Check sheet for the modelled part. Datum: model origin and axes. Units: mm. A direction names the side the tool comes from. Give positions to 0.01 mm unless a question says otherwise; leave off trailing zeros. Loops run counter-clockwise (first coordinate to the right, second up) from the corner with the lowest first, then second, coordinate; pieces in that order, holes last. Notation, with made-up numbers: (33, -11) -> (88, -11) arc R24 cw to (88, 12) -> close; hole circle Ø10 at (-26.75, -28.5). An arc over 180 degrees is marked (long way). Write each question's results on one line, items separated by ' | '. Start each with the question number.
1. Gauge pin test, flat ends, axial feed: pin 1 Ø6 at (y, z) = (21.5, 4) entering from +X; pin 2 Ø2.5 at (x, z) = (29, 7.5) entering from +Y; pin 3 Ø2 at (y, z) = (1, 10) entering from -X. Record the tip position at first contact, or that the pin passes through.
2. Cross-section at B-B on y = -11.25. Record the boundary of the cut face in (x, z), and give its area (3 significant figures).
3. Cross-section at C-C on x = 22.5. Record the boundary of the cut face in (y, z).
4. Cross-section at A-A on x = -40. Record the boundary of the cut face in (y, z), and give its area (3 significant figures).
5. Cross-section at D-D on y = -24. Record the boundary of the cut face in (x, z), and give its area (3 significant figures).
6. Tool access check on faces 5 (the face through (26, 1.25, 8)), 6 (the face through (27, 5.85, 5)), 7 (the face through (-40, -13, 2)), 8 (the face through (36, -13, 4)), 9 (the face through (42.747, -23.267, 7.379)). Record the directions out of +Z, -Z, +X, -X, +Y, -Y that give a thin tool (end or side, any length) a straight path to the whole face; none if there is none.
7. Mould release check, pull along X, two halves, no side actions. Record for faces 1 (the face through (34, -7, 7)), 2 (the face through (35.005, -15.662, 7.28)), 3 (the face through (1, -28, 7)), 4 (the face through (-25.08, 19.38, 7.4)): +X half, -X half, draft (parallel to the pull), parting line (faces both ways), or undercut.
8. Material ranges on L1, parallel to X at y = -10.5, z = 11.75; L2, parallel to Y at x = 22, z = 7.5; L3, parallel to Y at x = 0, z = 11.5, recorded low to high. Write a range as from..to.
from build123d import *

# Parameters (mm, degrees)
SKETCH1_R                                            = 21
BOSS_EXTRUDE1_DEPTH                                  = 15
SKETCH2_W                                            = 42.201264836
SKETCH2_H                                            = 2.5
CUT_EXTRUDE1_DEPTH                                   = 15
CUT_EXTRUDE2_DEPTH                                   = 15
CBORE_SLOT_FOR_M5_HEX_SOCKET_HEAD_CAP_SC_D           = 5.5
CBORE_SLOT_FOR_M5_HEX_SOCKET_HEAD_CAP_SC_CBORE_D     = 10
CBORE_SLOT_FOR_M5_HEX_SOCKET_HEAD_CAP_SC_CBORE_DEPTH = 5.4
CBORE_FOR_M5_HEX_SOCKET_HEAD_CAP_SCREW1_D            = 5.5
CBORE_FOR_M5_HEX_SOCKET_HEAD_CAP_SCREW1_DEPTH        = 10
CBORE_FOR_M5_HEX_SOCKET_HEAD_CAP_SCREW1_CBORE_D      = 9
CBORE_FOR_M5_HEX_SOCKET_HEAD_CAP_SCREW1_CBORE_DEPTH  = 5.4
CHAMFER1_SIZE                                        = 1
M4_TAPPED_HOLE1_D                                    = 3.3
M5_TAPPED_HOLE1_D                                    = 4.2
M5_TAPPED_HOLE1_DEPTH                                = 18
M5_TAPPED_HOLE1_TIP                                  = 1.2618073
CHAMFER2_SIZE                                        = 18
CHAMFER2_SIZE2                                       = 15.103793361
FILLET1_R                                            = 1


with BuildPart() as part:
    # Sketch1 → Boss-Extrude1 (new body)
    with BuildSketch(Plane.XY):
        Polygon((47, -28), (-47, -28), (-47, -13), (-34, -13), (-34, 27), (34, 27), (34, -13), (47, -13), align=None)
        Circle(SKETCH1_R, mode=Mode.SUBTRACT)
    extrude(amount=BOSS_EXTRUDE1_DEPTH)

    # Sketch2 → Cut-Extrude1 (cut)
    with BuildSketch(Plane.XY.offset(15)):
        with Locations((34, 0)):
            Rectangle(SKETCH2_W, SKETCH2_H)
    extrude(amount=-CUT_EXTRUDE1_DEPTH, mode=Mode.SUBTRACT)

    # Sketch3 → Cut-Extrude2 (cut)
    with BuildSketch(Plane.XY.offset(15)):
        Polygon((34, 27), (16, 27), (24, 11.25), (34, 11.25), align=None)
    extrude(amount=-CUT_EXTRUDE2_DEPTH, mode=Mode.SUBTRACT)

    # CBORE SLOT for M5 Hex Socket Head Cap Screw1 (through all)
    with Locations(Plane(origin=(0, -13, 0), x_dir=(1, 0, 0), z_dir=(0, 1, 0))):
        with Locations((-40, -7.5), (40, -7.5)):
            CounterBoreHole(CBORE_SLOT_FOR_M5_HEX_SOCKET_HEAD_CAP_SC_D / 2, CBORE_SLOT_FOR_M5_HEX_SOCKET_HEAD_CAP_SC_CBORE_D / 2, CBORE_SLOT_FOR_M5_HEX_SOCKET_HEAD_CAP_SC_CBORE_DEPTH)

    # CBORE for M5 Hex Socket Head Cap Screw1
    with Locations(Plane(origin=(29, 11.25, 7.5), x_dir=(0, 0, 1), z_dir=(0, 1, 0))):
        with Locations((0, 0)):
            CounterBoreHole(CBORE_FOR_M5_HEX_SOCKET_HEAD_CAP_SCREW1_D / 2, CBORE_FOR_M5_HEX_SOCKET_HEAD_CAP_SCREW1_CBORE_D / 2, CBORE_FOR_M5_HEX_SOCKET_HEAD_CAP_SCREW1_CBORE_DEPTH, depth=CBORE_FOR_M5_HEX_SOCKET_HEAD_CAP_SCREW1_DEPTH)

    # Chamfer1
    chamfer1_edges = [part.edges().sort_by_distance(p)[0] for p in [
        (47, -13, 7.5),
        (-47, -13, 7.5),
    ]]
    chamfer(chamfer1_edges, length=CHAMFER1_SIZE)

    # M4 Tapped Hole1 (through all)
    with Locations(Plane(origin=(-27, -21, 15), x_dir=(1, 0, 0), z_dir=(0, 0, 1))):
        with Locations((0, 0), (0, 20), (49, 0.741264898), (49, 9.75)):
            Hole(M4_TAPPED_HOLE1_D / 2)

    # M5 Tapped Hole1
    with Locations(Plane(origin=(29, -1.25, 7.5), x_dir=(1, 0, 0), z_dir=(0, 1, 0))):
        with Locations((0, 0)):
            Hole(M5_TAPPED_HOLE1_D / 2, depth=M5_TAPPED_HOLE1_DEPTH)
            with Locations((0, 0, -(M5_TAPPED_HOLE1_DEPTH + M5_TAPPED_HOLE1_TIP / 2))):  # 118° drill point
                Cone(0, M5_TAPPED_HOLE1_D / 2, M5_TAPPED_HOLE1_TIP, mode=Mode.SUBTRACT)

    # Chamfer2
    chamfer2_edges = [part.edges().sort_by_distance(p)[0] for p in [
        (-34, 27, 7.5),
    ]]
    chamfer2_side = [part.faces().sort_by_distance(p)[0] for p in [
        (-9, 27, 7.5),
    ]]
    chamfer(chamfer2_edges, length=CHAMFER2_SIZE, length2=CHAMFER2_SIZE2, reference=chamfer2_side[0])

    # Fillet1
    # the kernel refuses this fillet: 1 mm, written as the material it takes off along each edge
    with BuildSketch(Plane(origin=(47, -14, -1.035533906), x_dir=(0, -1, 0), z_dir=(0, 0, 1)), Plane(origin=(-47, -14, -1.035533906), x_dir=(0.7071067811865497, 0.7071067811865454, 0), z_dir=(0, 0, 1)), Plane(origin=(-46, -13, -1.035533906), x_dir=(1, 0, 0), z_dir=(0, 0, 1)), Plane(origin=(46, -13, -1.035533906), x_dir=(0.7071067811865455, -0.7071067811865497, 0), z_dir=(0, 0, 1))) as fillet1_piece_1:
        with BuildLine():
            CenterArc((FILLET1_R * 0.414213562373, -FILLET1_R), FILLET1_R, 90, 45)
            Line((-FILLET1_R * 0.292893218813, -FILLET1_R * 0.292893218813), (0, 0))
            Line((0, 0), (FILLET1_R * 0.414213562373, 0))
        make_face()
    extrude(amount=17.071067812, mode=Mode.SUBTRACT)
    with BuildSketch(Plane(origin=(-34, 11.896206639, -1.165769145), x_dir=(0, -1, 0), z_dir=(0, 0, 1))) as fillet1_piece_2:
        with BuildLine():
            CenterArc((FILLET1_R * 0.466307658155, FILLET1_R), FILLET1_R, 220, 50)
            Line((-FILLET1_R * 0.299736784964, FILLET1_R * 0.357212390313), (0, 0))
            Line((0, 0), (FILLET1_R * 0.466307658155, 0))
        make_face()
    extrude(amount=17.331538291, mode=Mode.SUBTRACT)
    with BuildSketch(Plane(origin=(-16, 27, -0.909925586), x_dir=(-0.7660444431189759, -0.6427876096865418, 0), z_dir=(0, 0, 1))) as fillet1_piece_3:
        with BuildLine():
            CenterArc((FILLET1_R * 0.363970234266, FILLET1_R), FILLET1_R, 230, 40)
            Line((-FILLET1_R * 0.27881737542, FILLET1_R * 0.233955556881), (0, 0))
            Line((0, 0), (FILLET1_R * 0.363970234266, 0))
        make_face()
    extrude(amount=16.819851171, mode=Mode.SUBTRACT)
    with BuildSketch(Plane(origin=(34, 11.25, 17.5), x_dir=(-1, 0, 0), z_dir=(0, 0, -1))) as fillet1_piece_4:
        with BuildLine():
            CenterArc((FILLET1_R, -FILLET1_R), FILLET1_R, 90, 90)
            Line((0, -FILLET1_R), (0, 0))
            Line((0, 0), (FILLET1_R, 0))
        make_face()
    extrude(amount=20, mode=Mode.SUBTRACT)
    with BuildSketch(Plane(origin=(16, 27, 16.534173147), x_dir=(-1, 0, 0), z_dir=(0, 0, -1))) as fillet1_piece_5:
        with BuildLine():
            CenterArc((FILLET1_R * 0.613669258853, -FILLET1_R), FILLET1_R, 90, 63.072322149)
            Line((-FILLET1_R * 0.27790960924, -FILLET1_R * 0.547134543191), (0, 0))
            Line((0, 0), (FILLET1_R * 0.613669258853, 0))
        make_face()
    extrude(amount=18.068346294, mode=Mode.SUBTRACT)


solid = part.part
Geometry says:
1) pin 1: x = 20.32 | pin 2: y = -19.76 | pin 3: x = -34
2) outline: (-34, 0) -> (-17.73, 0) -> (-17.73, 15) -> (-34, 15) -> close; (17.73, 0) -> (20.35, 0) -> (20.35, 15) -> (17.73, 15) -> close; (23.65, 0) -> (34, 0) -> (34, 15) -> (23.65, 15) -> close; hole circle Ø4.2 at (29, 7.5) | area: 425 mm^2
3) outline: (-28, 0) -> (-21.83, 0) -> (-21.83, 15) -> (-28, 15) -> close; (-18.69, 0) -> (-12.82, 0) -> (-12.82, 15) -> (-18.69, 15) -> close; (-9.68, 0) -> (-1.25, 0) -> (-1.25, 15) -> (-9.68, 15) -> close; (1.25, 0) -> (14.2, 0) -> (14.2, 15) -> (1.25, 15) -> close
4) outline: (-28, 0) -> (-13, 0) -> (-13, 2.5) -> (-18.4, 2.5) -> (-18.4, 4.75) -> (-28, 4.75) -> close; (-28, 10.25) -> (-18.4, 10.25) -> (-18.4, 12.5) -> (-13, 12.5) -> (-13, 15) -> (-28, 15) -> close | area: 118 mm^2
5) outline: (-47, 0) -> (47, 0) -> (47, 15) -> (-47, 15) -> close; hole circle Ø5.5 at (-40, 7.5); hole circle Ø5.5 at (40, 7.5) | area: 1,360 mm^2
6) face 5: +Z, -Z, +X | face 6: +Y | face 7: +Z, -Z, -X, +Y | face 8: +Z, -Z, +X, +Y | face 9: +Y, -Y
7) face 1: +X half | face 2: undercut | face 3: draft | face 4: -X half
8) L1: -34..-18.19, 18.19..20.53, 23.47..34 | L2: -28..-21.91, -18.61..-12.9, -9.6..-1.25, 1.25..15.19 | L3: -28..-21, 21..27
